Work out the finished part from the listing and answer in its coordinate system (mm). Face numbers are marked on the shaded views. Coordinates: 2 decimals unless noted, no trailing zeros. Order: outer loops, then holes, each group sorted by start corner. A loop starts at its lowest first (then second) coordinate and runs counter-clockwise, first axis right, second up. Notation, with made-up numbers: (18, 36.5) - (30, 36.5) arc R11 ccw to (30, 40.5) - close; hole circle Ø8 at (40, 28). An arc over 180 degrees is marked (long way). Answer as a JSON object with one key per item and string values. Group by question number.
1) Each of these flat-tipped pins is pushed along its axis until it touches: P1, Ø6, axis at y = 10, z = 23.5, coming from the +X side; P2, Ø4, axis at x = 11, z = 16, coming from the +Y side. Where does it stop, or does it pass through?
2) Find the intervals of material crossed by line 1 along X through (y, z) = (10, 30); line 2 along X through (y, z) = (17.5, 45), in increasing order.
3) Section A-A (y = 10) is taken. Give the vertices of the cut face in (x, z), plus the area to 3 significant figures.
4) The mould has two halves that part along X. Classify the marked faces 1, 2 and 3: released by +X, released by -X, zero draft, split by the parting line, or undercut.
from build123d import *

# Parameters (mm, degrees)
SKETCH_1_R      = 2.5
EXTRUDE_1_DEPTH = 57
FILLET_1_R      = 1.5
FILLET_2_R      = 1.5
FILLET_3_R      = 1.5
FILLET_4_R      = 1.5
FILLET_5_R      = 0.5
FILLET_6_R      = 0.5
FILLET_7_R      = 0.5
FILLET_8_R      = 0.5
FILLET_9_R      = 0.5
FILLET_10_R     = 0.5
FILLET_11_R     = 0.5
FILLET_12_R     = 0.5


with BuildPart() as part:
    # 草图1 → 凸台-拉伸1 (new body)
    with BuildSketch(Plane.XY):
        Polygon((0, 6.9), (0, 0), (6.9, 0), (6.9, 1.8), (4.5, 1.8), (4.5, 3.227207794), (7.372792206, 6.1), (12.627207794, 6.1), (15.5, 3.227207794), (15.5, 1.8), (13.1, 1.8), (13.1, 0), (20, 0), (20, 6.9), (18.2, 6.9), (18.2, 4.5), (16.772792206, 4.5), (13.9, 7.372792206), (13.9, 12.627207794), (16.772792206, 15.5), (18.2, 15.5), (18.2, 13.1), (20, 13.1), (20, 20), (13.1, 20), (13.1, 18.2), (15.5, 18.2), (15.5, 16.772792206), (12.627207794, 13.9), (7.372792206, 13.9), (4.5, 16.772792206), (4.5, 18.2), (6.9, 18.2), (6.9, 20), (0, 20), (0, 13.1), (1.8, 13.1), (1.8, 15.5), (3.227207794, 15.5), (6.1, 12.627207794), (6.1, 7.372792206), (3.227207794, 4.5), (1.8, 4.5), (1.8, 6.9), align=None)
        with Locations(Location((10, 10, 0), (0, 0, 180))):
            Circle(SKETCH_1_R, mode=Mode.SUBTRACT)
    extrude(amount=EXTRUDE_1_DEPTH)

    # 圆角1
    fillet_1_edges = [part.edges().sort_by_distance(p)[0] for p in [
        (20, 20, 28.5),
    ]]
    fillet(fillet_1_edges, radius=FILLET_1_R)

    # 圆角2
    fillet_2_edges = [part.edges().sort_by_distance(p)[0] for p in [
        (0, 20, 28.5),
    ]]
    fillet(fillet_2_edges, radius=FILLET_2_R)

    # 圆角3
    fillet_3_edges = [part.edges().sort_by_distance(p)[0] for p in [
        (0, 0, 28.5),
    ]]
    fillet(fillet_3_edges, radius=FILLET_3_R)

    # 圆角4
    fillet_4_edges = [part.edges().sort_by_distance(p)[0] for p in [
        (20, 0, 28.5),
    ]]
    fillet(fillet_4_edges, radius=FILLET_4_R)

    # 圆角5
    fillet_5_edges = [part.edges().sort_by_distance(p)[0] for p in [
        (13.1, 20, 28.5),
    ]]
    fillet(fillet_5_edges, radius=FILLET_5_R)

    # 圆角6
    fillet_6_edges = [part.edges().sort_by_distance(p)[0] for p in [
        (6.9, 20, 28.5),
    ]]
    fillet(fillet_6_edges, radius=FILLET_6_R)

    # 圆角7
    fillet_7_edges = [part.edges().sort_by_distance(p)[0] for p in [
        (0, 13.1, 28.5),
    ]]
    fillet(fillet_7_edges, radius=FILLET_7_R)

    # 圆角8
    fillet_8_edges = [part.edges().sort_by_distance(p)[0] for p in [
        (0, 6.9, 28.5),
    ]]
    fillet(fillet_8_edges, radius=FILLET_8_R)

    # 圆角9
    fillet_9_edges = [part.edges().sort_by_distance(p)[0] for p in [
        (6.9, 0, 28.5),
    ]]
    fillet(fillet_9_edges, radius=FILLET_9_R)

    # 圆角10
    fillet_10_edges = [part.edges().sort_by_distance(p)[0] for p in [
        (13.1, 0, 28.5),
    ]]
    fillet(fillet_10_edges, radius=FILLET_10_R)

    # 圆角11
    fillet_11_edges = [part.edges().sort_by_distance(p)[0] for p in [
        (20, 13.1, 28.5),
    ]]
    fillet(fillet_11_edges, radius=FILLET_11_R)

    # 圆角12
    fillet_12_edges = [part.edges().sort_by_distance(p)[0] for p in [
        (20, 6.9, 28.5),
    ]]
    fillet(fillet_12_edges, radius=FILLET_12_R)


solid = part.part
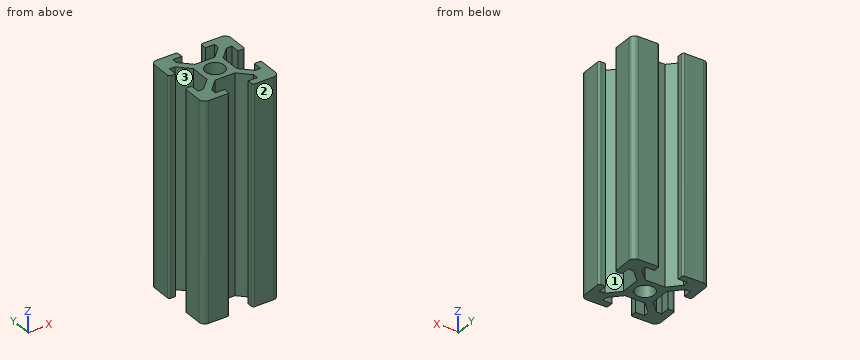
Report:
{
 "1": {"P1": "stops at x = 14.27", "P2": "stops at y = 14.27"},
 "2": {"line 1": "x = 6.1 to 7.5, 12.5 to 13.9", "line 2": "x = 0 to 4.5, 15.5 to 20"},
 "3": {"outline": "(6.1, 0) - (7.5, 0) - (7.5, 57) - (6.1, 57) - close; (12.5, 0) - (13.9, 0) - (13.9, 57) - (12.5, 57) - close", "area": "160 mm²"},
 "4": {"face 1": "undercut", "face 2": "zero draft", "face 3": "undercut"}
}
